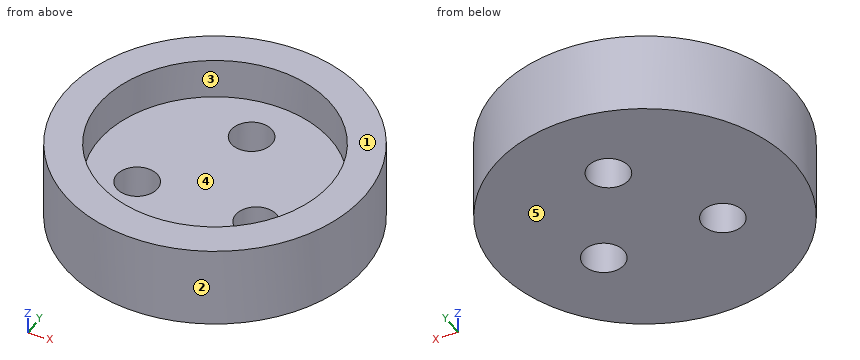
```python
from build123d import *

# Parameters (mm, degrees)
ESQUISSE1_R        = 11
ESQUISSE1_R_2      = 1.5
BOSS_EXTRU_1_DEPTH = 3
ESQUISSE2_R        = 11
ESQUISSE2_R_2      = 8.5
BOSS_EXTRU_2_DEPTH = 3


with BuildPart() as part:
    # Esquisse1 → Boss.-Extru.1 (new body)
    with BuildSketch(Plane.XY):
        Circle(ESQUISSE1_R)
        with Locations((0, 5)):
            Circle(ESQUISSE1_R_2, mode=Mode.SUBTRACT)
        with Locations((4.330127019, -2.5)):
            Circle(ESQUISSE1_R_2, mode=Mode.SUBTRACT)
        with Locations((-4.330127019, -2.5)):
            Circle(ESQUISSE1_R_2, mode=Mode.SUBTRACT)
    extrude(amount=BOSS_EXTRU_1_DEPTH)

    # Esquisse2 → Boss.-Extru.2 (add)
    with BuildSketch(Plane.XY.offset(3)):
        Circle(ESQUISSE2_R)
        Circle(ESQUISSE2_R_2, mode=Mode.SUBTRACT)
    extrude(amount=BOSS_EXTRU_2_DEPTH)


solid = part.part
```
Geometry check sheet. Reference: the model listing, model coordinates, mm. Face numbers are marked on the shaded views. A direction names the side the tool comes from. Coordinates: 2 decimals unless noted, no trailing zeros. Order: outer loops, then holes, each group sorted by start corner. A loop starts at its lowest first (then second) coordinate and runs counter-clockwise, first axis right, second up.
Q1. Depth check by flat-ended pin: pin 1 Ø3 at (y, z) = (5.5, 2.5) entering from -X; pin 2 Ø1 at (y, z) = (-1, 3) entering from -X; pin 3 Ø4 at (x, y) = (0, 5) entering from +Z. Enter the tip coordinate at first touch or a pass-through.
Reply:
pin 1: stops at x = -10.25
pin 2: stops at x = -10.99
pin 3: stops at z = 3
Q2. Sectioned sample at D-D on z = 4.85. Record the cut outline in (x, y), and give its area (3 significant figures).
Reply:
outline: circle Ø22 at (0, 0); hole circle Ø17 at (0, 0)
area: 153 mm2
Q3. Sectioned sample at A-A on x = 0. Record the cut outline in (y, z), and give its area (3 significant figures).
Reply:
outline: (-11, 0) - (3.5, 0) - (3.5, 3) - (-8.5, 3) - (-8.5, 6) - (-11, 6) - close; (6.5, 0) - (11, 0) - (11, 6) - (8.5, 6) - (8.5, 3) - (6.5, 3) - close
area: 72.0 mm2
Q4. Thickness scan on probe 1 along Y at (x, z) = (0, 5.2); probe 2 along Y at (x, z) = (0, 1); probe 3 along Z at (x, y) = (6, -2.5). Record the ranges inside material, lowest first.
Reply:
probe 1: y = -11 to -8.5, 8.5 to 11
probe 2: y = -11 to 3.5, 6.5 to 11
probe 3: z = 0 to 3
Q5. Sectioned sample at B-B on y = 0. Record the cut outline in (x, z).
Reply:
outline: (-11, 0) - (11, 0) - (11, 6) - (8.5, 6) - (8.5, 3) - (-8.5, 3) - (-8.5, 6) - (-11, 6) - close
Q6. Tool access check on the marked faces 4 and 5. Record the directions out of +Z, -Z, +X, -X, +Y, -Y that give a thin tool (end or side, any length) a straight path to the whole face; none if there is none.
Reply:
face 4: +Z
face 5: -Z, +X, -X, +Y, -Y
Q7. Sectioned sample at C-C on y = 5. Record the cut outline in (x, z), and give its area (3 significant figures).
Reply:
outline: (-9.8, 0) - (-1.5, 0) - (-1.5, 3) - (-6.87, 3) - (-6.87, 6) - (-9.8, 6) - close; (1.5, 0) - (9.8, 0) - (9.8, 6) - (6.87, 6) - (6.87, 3) - (1.5, 3) - close
area: 67.3 mm2
Q8. Draft check along X on the marked faces 1, 2 and 3. Enter one of: released by +X, released by -X, zero draft, split by the parting line, or undercut.
Reply:
face 1: zero draft
face 2: split by the parting line
face 3: undercut
